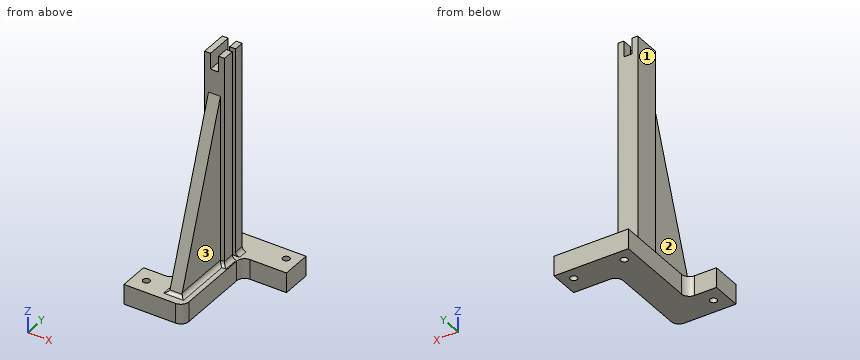
```python
from build123d import *

# Parameters (mm, degrees)
SKETCH1_R           = 1.75
BOSS_EXTRUDE1_DEPTH = 10
BOSS_EXTRUDE2_DEPTH = 105
RIB1_REACH          = 134.949
SKETCH3_WALL_W      = 358.03606807
SKETCH3_WALL_H      = 6
FILLET1_R           = 4
FILLET2_R           = 2
SKETCH4_W           = 4
SKETCH4_H           = 13.56
CUT_EXTRUDE1_DEPTH  = 8


with BuildPart() as part:
    # Sketch1 → Boss-Extrude1 (new body)
    with BuildSketch(Plane.XY):
        Polygon((0, 0), (0, 15), (15, 15), (15, 59.64), (52.39, 59.64), (52.39, 44.64), (30, 44.64), (30, 0), align=None)
        with Locations((6.39, 7.5)):
            Circle(SKETCH1_R, mode=Mode.SUBTRACT)
        with Locations((21, 53.64)):
            Circle(SKETCH1_R, mode=Mode.SUBTRACT)
        with Locations((46.39, 53.64)):
            Circle(SKETCH1_R, mode=Mode.SUBTRACT)
    extrude(amount=BOSS_EXTRUDE1_DEPTH)

    # Sketch2 → Boss-Extrude2 (add)
    with BuildSketch(Plane.XY.offset(10)):
        Polygon((27.5, 48.64), (17.5, 48.64), (17.5, 35.08), (27.5, 35.08), (27.5, 41.08), (22.477989852, 41.08), (22.477989852, 43.64), (27.5, 43.64), align=None)
    extrude(amount=BOSS_EXTRUDE2_DEPTH)

    # Sketch3 wall → Rib1 (add, up to next)
    with BuildSketch(Plane(origin=(22.5, 20.08, 52.5), x_dir=(0, 0.332820117735, 0.942990333583), z_dir=(0, -0.942990333583, 0.332820117735)), mode=Mode.PRIVATE) as rib1_sk1:
        Rectangle(SKETCH3_WALL_W, SKETCH3_WALL_H)
    rib1_tool1 = extrude(rib1_sk1.sketch, amount=-RIB1_REACH, mode=Mode.PRIVATE) - part.part
    add(rib1_tool1.solids().sort_by_distance((22.5, 20.08, 52.5))[0])

    # Fillet1
    fillet1_edges = [part.edges().sort_by_distance(p)[0] for p in [
        (15, 15, 5),
        (30, 44.64, 5),
        (30, 0, 5),
    ]]
    fillet(fillet1_edges, radius=FILLET1_R)

    # Fillet2
    fillet2_edges = [part.edges().sort_by_distance(p)[0] for p in [
        (27.5, 46.14, 10),
        (27.5, 38.08, 10),
        (26.5, 35.08, 10),
        (25.5, 20.08, 10),
        (19.5, 20.08, 10),
        (18.5, 35.08, 10),
        (17.5, 41.86, 10),
        (22.5, 5.08, 10),
    ]]
    fillet(fillet2_edges, radius=FILLET2_R)

    # Sketch4 → Cut-Extrude1 (cut)
    with BuildSketch(Plane.XY.offset(115)):
        with Locations((22.5, 41.86)):
            Rectangle(SKETCH4_W, SKETCH4_H)
    extrude(amount=-CUT_EXTRUDE1_DEPTH, mode=Mode.SUBTRACT)


solid = part.part
```
Work out the finished part from the listing and answer in its coordinate system (mm). Face numbers are marked on the shaded views. A direction names the side the tool comes from. Give positions to 0.01 mm unless a question says otherwise; leave off trailing zeros. Loops run counter-clockwise (first coordinate to the right, second up) from the corner with the lowest first, then second, coordinate; pieces in that order, holes last. Notation, with made-up numbers: (-15, 32.5) -> (29, 32.5) arc R9 ccw to (29, 47.5) -> close; hole circle Ø3 at (13, -32.5). An arc over 180 degrees is marked (long way). Write item = value, one per line. Start each with the question number.
(1) Find section B-B on y = 53.64. Give the vertices of the cut face in (x, z), and give its area (3 significant figures).
(2) Which of the six approach directions +Z, -Z, +X, -X, +Y, -Y give full straight-line access (tool end or side, diameter ignored) to the marked faces 1, 2 and 3?
(3) Find section C-C on y = 37.5. Give the vertices of the cut face in (x, z).
(4) Find section A-A on x = 6.39. Give the vertices of the cut face in (y, z).
(5) Given pin 1 Ø3 at (x, y) = (40.5, 46.5) entering from +Z; pin 2 Ø15.5 at (x, z) = (21.5, 46) entering from +Y; pin 3 Ø1.8 at (y, z) = (39, 88.5) entering from +X, each flat-ended and moving along its own axis, determine where each tip first touches the part or whether it passes through.
(6) Find section D-D on y = 7.5. Give the vertices of the cut face in (x, z).
(7) Find the intervals of material crossed by probe 1 along Y at (x, z) = (6.39, 3.25); probe 2 along X at (y, z) = (53, 2); probe 3 along Y at (x, z) = (21, 7), in increasing order. Write a range as from..to.
From the geometry:
q1.outline = (15, 0) -> (19.25, 0) -> (19.25, 10) -> (15, 10) -> close; (22.75, 0) -> (44.64, 0) -> (44.64, 10) -> (22.75, 10) -> close; (48.14, 0) -> (52.39, 0) -> (52.39, 10) -> (48.14, 10) -> close
q1.area = 304 mm^2
q2.face_1 = +Z, -X, +Y, -Y
q2.face_2 = +Z, -X, -Y
q2.face_3 = +Z, +X, -Y
q3.outline = (15, 0) -> (30, 0) -> (30, 10) -> (29.5, 10) arc R2 cw to (27.5, 12) -> (27.5, 115) -> (24.5, 115) -> (24.5, 107) -> (20.5, 107) -> (20.5, 115) -> (17.5, 115) -> (17.5, 12) arc R2 cw to (15.5, 10) -> (15, 10) -> close
q4.outline = (0, 0) -> (5.75, 0) -> (5.75, 10) -> (0, 10) -> close; (9.25, 0) -> (15, 0) -> (15, 10) -> (9.25, 10) -> close
q5.pin_1 = 10
q5.pin_2 = 48.64
q5.pin_3 = 27.5
q6.outline = (0, 0) -> (4.64, 0) -> (4.64, 10) -> (0, 10) -> close; (8.14, 0) -> (30, 0) -> (30, 10) -> (27.5, 10) arc R2 cw to (25.5, 12) -> (25.5, 16.86) -> (19.5, 16.86) -> (19.5, 12) arc R2 cw to (17.5, 10) -> (8.14, 10) -> close
q7.probe_1 = 0..5.75, 9.25..15
q7.probe_2 = 15..19.37, 22.63..44.76, 48.02..52.39
q7.probe_3 = 0..51.89, 55.39..59.64
